Read the model definition and answer for the solid it produces. Units are mm, in the model's axes. Give positions to 0.01 mm unless a question says otherwise; leave off trailing zeros. Write each loop counter-clockwise with the first axis right and the second up, starting at its lowest first coordinate (ties: lowest second). Pieces come first, ordered by that corner, then holes. Notation, with made-up numbers: (-39.75, 73) -> (-8.75, 73) arc R22 ccw to (-8.75, 93) -> close; hole circle Ø8 at (-13.75, 26). An arc over 180 degrees is marked (long way). Use a Markdown table: item, result.
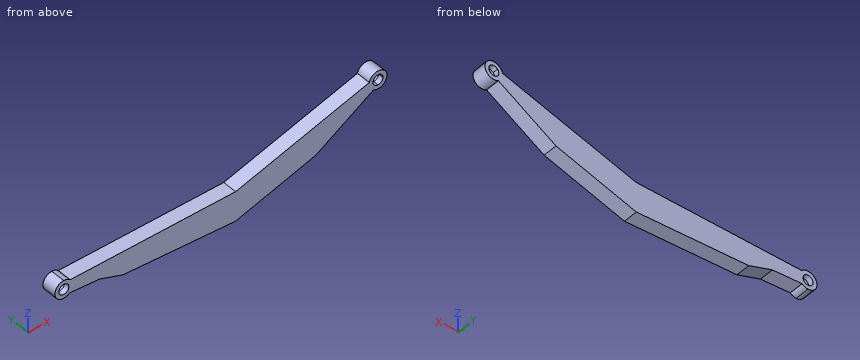
from build123d import *

# Parameters (mm, degrees)
F1_DEPTH = 25.4


with BuildPart() as f1:
    # F0 (on Front) → F1 (new body)
    with BuildSketch(Plane.XZ):
        with BuildLine():
            ThreePointArc((75.5846782372, 0), (74.4064598557, 6.0016860181), (71.0466958676, 11.1125))
            Line((71.0466958676, 11.1125), (59.7096782372, 11.1125))
            Line((59.7096782372, 11.1125), (59.7096782372, 8.89))
            ThreePointArc((59.7096782372, 8.89), (65.995857522, 6.2861792847), (68.5996782372, 0))
            ThreePointArc((68.5996782372, 0), (65.995857522, -6.2861792847), (59.7096782372, -8.89))
            Line((59.7096782372, -8.89), (59.7096782372, -11.1125))
            Line((59.7096782372, -11.1125), (70.2693648091, -11.8536342319))
            ThreePointArc((70.2693648091, -11.8536342319), (74.195026858, -6.4954060948), (75.5846782372, 0))
        make_face()
        with BuildLine():
            ThreePointArc((71.0466958676, 11.1125), (65.8580392994, 14.636026826), (59.7096782372, 15.875))
            Line((59.7096782372, 15.875), (59.7096782372, 11.1125))
            Line((59.7096782372, 11.1125), (71.0466958676, 11.1125))
        make_face()
        with BuildLine():
            Line((59.7096782372, 11.1125), (59.7096782372, 15.875))
            ThreePointArc((59.7096782372, 15.875), (43.8346782372, 0), (59.7096782372, -15.875))
            Line((59.7096782372, -15.875), (59.7096782372, -11.1125))
            Line((59.7096782372, -11.1125), (59.7096782372, -8.89))
            ThreePointArc((59.7096782372, -8.89), (50.8196782372, 0), (59.7096782372, 8.89))
            Line((59.7096782372, 8.89), (59.7096782372, 11.1125))
        make_face()
        with BuildLine():
            Line((59.7096782372, -11.1125), (59.7096782372, -15.875))
            ThreePointArc((59.7096782372, -15.875), (65.3594207786, -14.8356339337), (70.2693648091, -11.8536342319))
            Line((70.2693648091, -11.8536342319), (59.7096782372, -11.1125))
        make_face()
        with BuildLine():
            Line((364.5096782372, 11.1125), (71.0466958676, 11.1125))
            ThreePointArc((71.0466958676, 11.1125), (74.4064598557, 6.0016860181), (75.5846782372, 0))
            ThreePointArc((75.5846782372, 0), (74.195026858, -6.4954060948), (70.2693648091, -11.8536342319))
            Line((70.2693648091, -11.8536342319), (123.0538541683, -15.5583267636))
            Line((123.0538541683, -15.5583267636), (164.9836269965, -30.31287354))
            Line((164.9836269965, -30.31287354), (364.5096782372, -41.5203937454))
            Line((364.5096782372, -41.5203937454), (364.5096782372, 11.1125))
        make_face()
        with BuildLine():
            Line((528.8047229938, 57.9100469965), (364.5096782372, 11.1125))
            Line((364.5096782372, 11.1125), (364.5096782372, -41.5203937454))
            Line((364.5096782372, -41.5203937454), (506.9307684898, 0))
            Line((506.9307684898, 0), (609.0909272925, 61.5520499979))
            ThreePointArc((609.0909272925, 61.5520499979), (602.6243965326, 68.918336487), (601.716619668, 78.6781591222))
            Line((601.716619668, 78.6781591222), (528.8047229938, 57.9100469965))
        make_face()
        with BuildLine():
            Line((610.6760785802, 81.2301575719), (601.716619668, 78.6781591222))
            ThreePointArc((601.716619668, 78.6781591222), (602.6243965326, 68.918336487), (609.0909272925, 61.5520499979))
            Line((609.0909272925, 61.5520499979), (616.9867526025, 66.3093275899))
            ThreePointArc((616.9867526025, 66.3093275899), (609.017363859, 71.7336687669), (610.6760785802, 81.2301575719))
        make_face()
        with BuildLine():
            ThreePointArc((633.0801535113, 75.196644454), (618.956602945, 90.9747321037), (601.716619668, 78.6781591222))
            Line((601.716619668, 78.6781591222), (610.6760785802, 81.2301575719))
            ThreePointArc((610.6760785802, 81.2301575719), (620.4446460535, 83.4753996786), (626.0951535113, 75.196644454))
            ThreePointArc((626.0951535113, 75.196644454), (623.4136362535, 68.8337172943), (616.9867526025, 66.3093275899))
            Line((616.9867526025, 66.3093275899), (609.0909272925, 61.5520499979))
            ThreePointArc((609.0909272925, 61.5520499979), (625.0537930041, 61.3975690099), (633.0801535113, 75.196644454))
        make_face()
    extrude(amount=F1_DEPTH)

    # F3 (on offset) → F4 (revolve, cut)
    with BuildSketch(Plane.XZ.offset(12.7)):
        with BuildLine():
            Line((59.7096782372, 0), (59.7096782372, -9.525))
            ThreePointArc((59.7096782372, -9.525), (69.2346782372, 0), (59.7096782372, 9.525))
            Line((59.7096782372, 9.525), (59.7096782372, 0))
        make_face()
    revolve(axis=Axis((59.7096782372, -12.7, 0), (0, 0, -1)), mode=Mode.SUBTRACT)

    # F3 (on offset) → F5 (revolve, cut)
    with BuildSketch(Plane.XZ.offset(12.7)):
        with BuildLine():
            Line((617.2051535113, 75.196644454), (617.2051535113, 65.671644454))
            ThreePointArc((617.2051535113, 65.671644454), (626.7301535113, 75.196644454), (617.2051535113, 84.721644454))
            Line((617.2051535113, 84.721644454), (617.2051535113, 75.196644454))
        make_face()
    revolve(axis=Axis((617.2051535113, -12.7, 75.196644454), (0, 0, -1)), mode=Mode.SUBTRACT)


solid = f1.part
Item 1: A cutting plane is placed at B-B (z = -23). Give the vertices of the cut face in (x, y), then the cut area to 3 significant figures.
Return value:
| item | result |
|---|---|
| outline | (144.2, -25.4) -> (428.04, -25.4) -> (428.04, 0) -> (144.2, 0) -> close |
| area | 7,210 mm^2 |
Item 2: Each of these flat-tipped pins is pushed along its axis until it touches: P1, Ø1, axis at y = -22, z = 66.5, coming from the +X side; P2, Ø1.5, axis at x = 364, z = 12.5, coming from the -Y side; P3, Ø3, axis at y = -9.5, z = -14.5, coming from the -X side; P4, Ø12.5, axis at x = 215.5, y = -12, coming from the +Z side. Where does it stop, or does it pass through?
Return value:
| item | result |
|---|---|
| P1 | x = 630.8 |
| P2 | through |
| P3 | x = 50.6 |
| P4 | z = 11.11 |
Item 3: A cutting plane is placed at A-A (x = 519.5). Give the vertices of the cut face in (y, z).
Return value:
| item | result |
|---|---|
| outline | (-25.4, 7.57) -> (0, 7.57) -> (0, 55.26) -> (-25.4, 55.26) -> close |
Item 4: Straight lines are drawn through the part: line 1 along Z through (x, y) = (112, -14.75); line 2 along X through (y, z) = (-7, 2); line 3 along Z through (x, y) = (329, -16.5). For each, find the intervals that lie inside material, in ascending order. Write a range as [from, to].
Return value:
| item | result |
|---|---|
| line 1 | [-14.78, 11.11] |
| line 2 | [43.96, 51.05], [68.37, 510.25] |
| line 3 | [-39.53, 11.11] |
